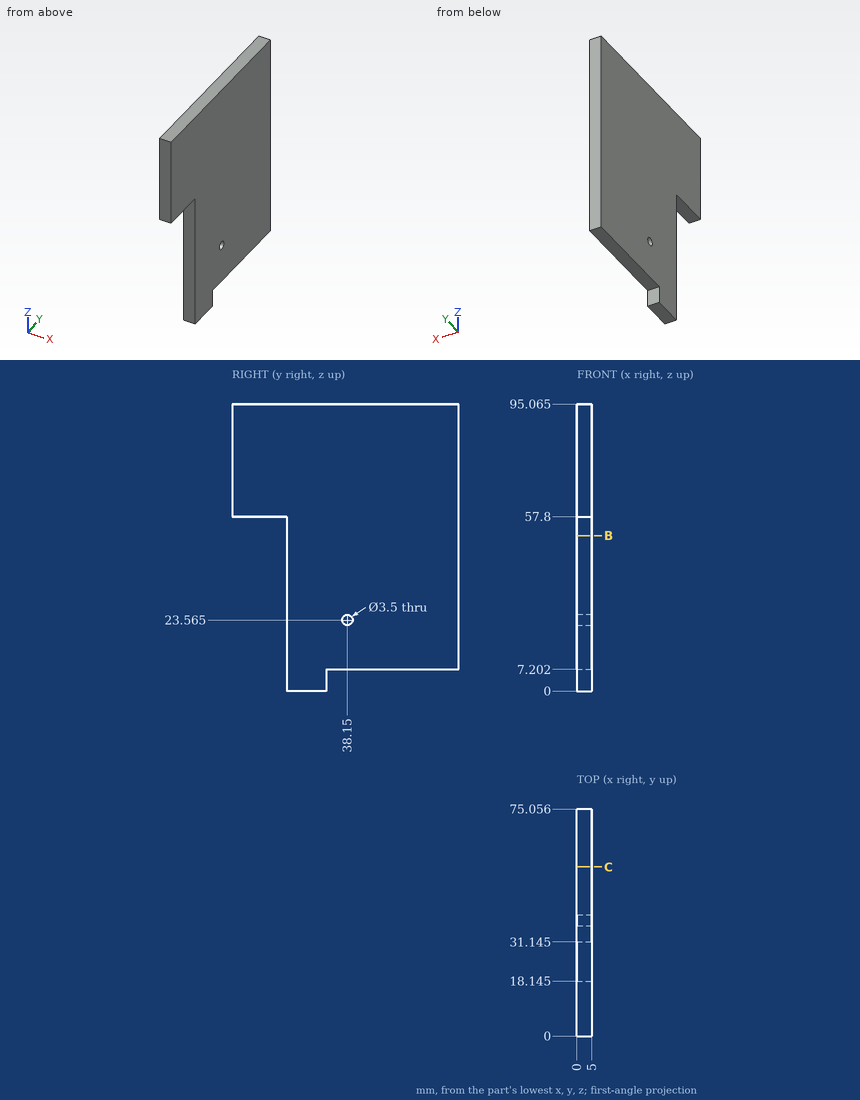
Study the drawing (mm; zero at the part's minimum x, y, z) and answer. Give positions to 0.01 mm unless a question says otherwise; leave off trailing zeros. Loops run counter-clockwise (first coordinate to the right, second up) from the corner with the lowest first, then second, coordinate; pieces in that order, holes last. Notation, with made-up numbers: (-23.5, 43) - (4.5, 43) arc R19 ccw to (4.5, 59) - close; hole circle Ø1 at (-24.5, 11.25). An arc over 180 degrees is marked (long way). Answer in a Markdown table with one row per item. Add a question column.
Q1. The part is cut by section C-C (y = 56). Determine the outline of the cut face in (x, z) (1 decimal), and give its area (3 significant figures).
Q2. Each of these flat-tipped pins is pushed along its axis until it touches: P1, Ø2.5, axis at x = 3, z = 3.5, coming from the +Y side (1 decimal); P2, Ø1, axis at x = 4, z = 16.5, coming from the -Y side (1 decimal). Where does it stop, or does it pass through?
Q3. Consider line 1 along Z through (x, y) = (0.3, 7) (1 decimal); line 2 along Y through (x, z) = (4.2, 13.5) (1 decimal); line 3 along Z through (x, y) = (2.3, 43.5) (1 decimal). Determine where each line is inside the solid, lowest interval first.
Q4. The part is cut by section B-B (z = 51.5). Determine the outline of the cut face in (x, y) (1 decimal).
Solution:
| question | item | result |
|---|---|---|
| 1 | outline | (0, 7.2) - (5, 7.2) - (5, 95.1) - (0, 95.1) - close |
| 1 | area | 439 mm² |
| 2 | P1 | stops at y = 31.1 |
| 2 | P2 | stops at y = 18.1 |
| 3 | line 1 | z = 57.8 to 95.1 |
| 3 | line 2 | y = 18.1 to 75.1 |
| 3 | line 3 | z = 7.2 to 95.1 |
| 4 | outline | (0, 18.1) - (5, 18.1) - (5, 75.1) - (0, 75.1) - close |
